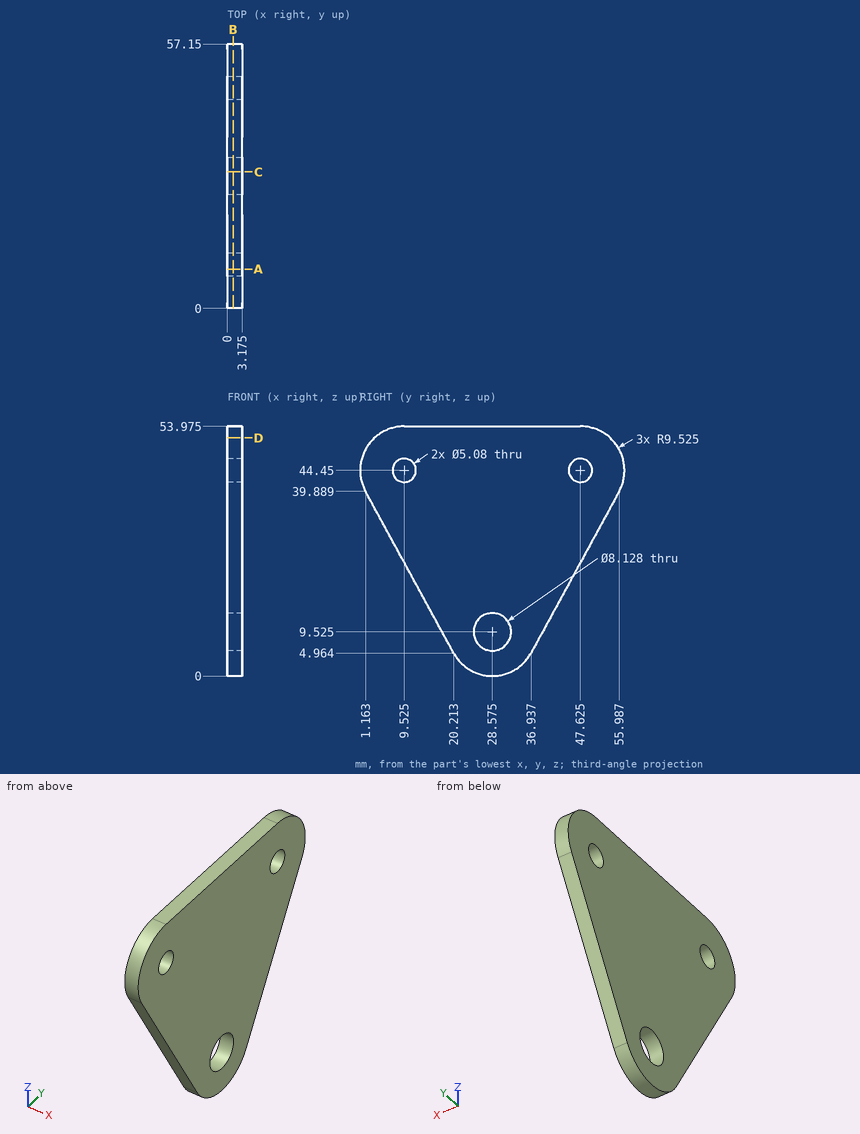
Check sheet for the drawn part. Datum: minimum x, y, z corner. Units: mm. Give positions to 0.01 mm unless a question says otherwise; leave off trailing zeros. Order: outer loops, then holes, each group sorted by start corner. A loop starts at its lowest first (then second) coordinate and runs counter-clockwise, first axis right, second up. Notation, with made-up numbers: (-24.75, 12) - (17.25, 12) arc R22 cw to (17.25, 31) - close; hole circle Ø8 at (-40, 60). An arc over 180 degrees is marked (long way). Write item = value, one per line. Start each with the question number.
1) Scan lines: L1, parallel to Y at x = 0.2, z = 43; L2, parallel to Z at x = 2.5, y = 26.5 (1 decimal); L3, parallel to Z at x = 1, y = 31.5 (1 decimal). Record each from-to range of solid material in increasing order.
2) Section check A-A (y = 8.5). Enter the section's corners in (x, z) (3 decimals).
3) Section check B-B (x = 1.2). Enter the section's corners in (y, z) (3 decimals), then the cut area to 3 significant figures.
4) Section check C-C (y = 29.5). Enter the section's corners in (x, z) (1 decimal), then the cut area to 3 significant figures.
5) Section check D-D (z = 51.5). Enter the section's corners in (x, y) (3 decimals), then the cut area to 3 significant figures.
6) Gauge pin test, flat ends, axial feed: pin 1 Ø6.5 at (y, z) = (28.58, 9.53) entering from -X; pin 2 Ø1.5 at (x, z) = (2, 40) entering from -Y. Record the tip position at first contact, or that the pin passes through.
Geometry check:
q1.L1 = 0.11 to 7.44, 11.61 to 45.54, 49.71 to 57.04
q1.L2 = 0.2 to 6, 13 to 54
q1.L3 = 0.5 to 6.7, 12.3 to 54
q2.outline = (0, 26.438) - (3.175, 26.438) - (3.175, 42.126) - (0, 42.126) - close; (0, 46.774) - (3.175, 46.774) - (3.175, 53.92) - (0, 53.92) - close
q3.outline = (1.163, 39.889) - (20.213, 4.964) arc R9.525 ccw to (36.937, 4.964) - (55.987, 39.889) arc R9.525 ccw to (47.625, 53.975) - (9.525, 53.975) arc R9.525 ccw to start; hole circle Ø5.08 at (9.525, 44.45); hole circle Ø8.128 at (28.575, 9.525); hole circle Ø5.08 at (47.625, 44.45)
q3.area = 1,980 mm2
q4.outline = (0, 0) - (3.2, 0) - (3.2, 5.6) - (0, 5.6) - close; (0, 13.5) - (3.2, 13.5) - (3.2, 54) - (0, 54) - close
q4.area = 146 mm2
q5.outline = (0, 3.12) - (3.175, 3.12) - (3.175, 54.03) - (0, 54.03) - close
q5.area = 162 mm2
q6.pin_1 = through
q6.pin_2 = 0.75
